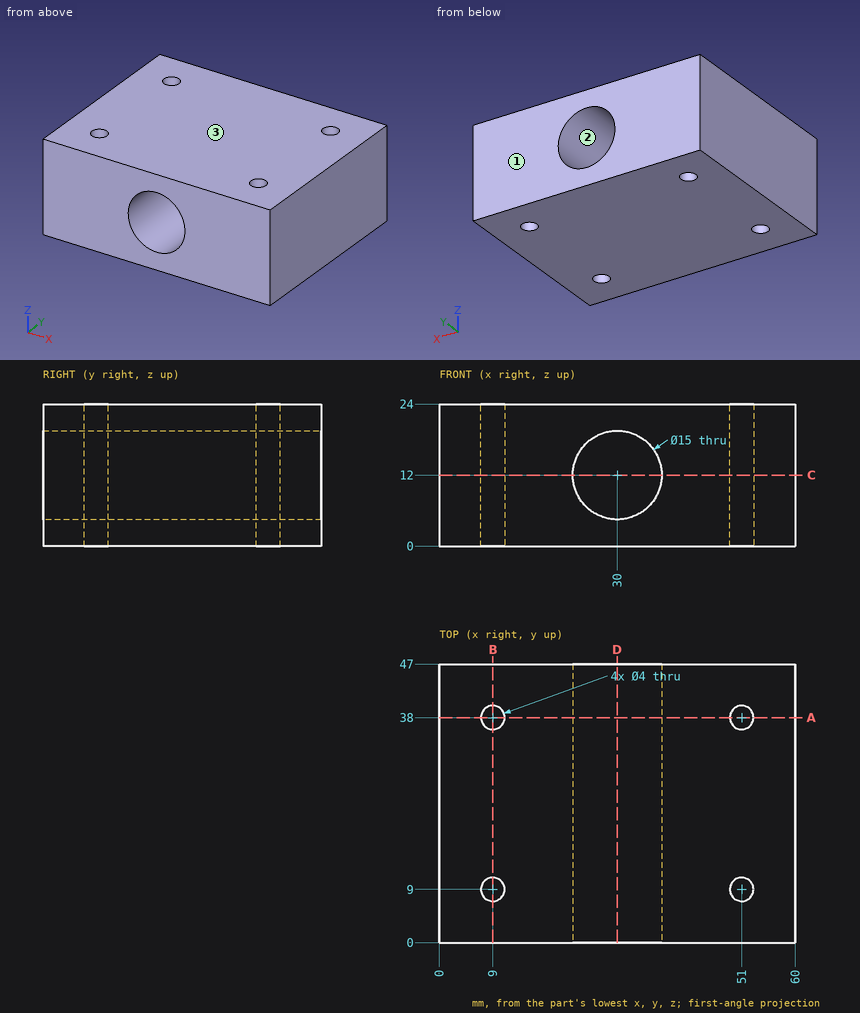
Input: dimensioned drawing with shaded views. Units: mm. Origin: part minimum x, y, z. Round coordinates to 2 decimals unless told otherwise and drop trailing zeros. Loops run counter-clockwise (first coordinate to the right, second up) from the corner with the lowest first, then second, coordinate; pieces in that order, holes last. Notation, with made-up numbers: M 66.25,88.5 L 115.25,88.5 A16 ccw 115.25,99.5 Z; hole C 9,8.5 d10. An arc over 180 degrees is marked long. One line per question, with ' | ' between items.
(1) Cut plane D-D on x = 30. Return the cut outline in (y, z), plus the area to 3 significant figures.
Check result:
outline: M 0,0 L 47,0 L 47,4.5 L 0,4.5 Z; M 0,19.5 L 47,19.5 L 47,24 L 0,24 Z | area: 423 mm2
(2) Cut plane C-C on z = 12. Return the cut outline in (x, y).
Check result:
outline: M 0,0 L 22.5,0 L 22.5,47 L 0,47 Z; M 37.5,0 L 60,0 L 60,47 L 37.5,47 Z; hole C 9,9 d4; hole C 9,38 d4; hole C 51,9 d4; hole C 51,38 d4
(3) Pull-direction query (Z, two-part tool) for the marked faces 1, 2 and 3; classes: +Z half, -Z half, draft (parallel to the pull), parting line (faces both ways), or undercut.
Check result:
face 1: draft | face 2: undercut | face 3: +Z half
(4) Contact query for a flat-ended pin moving along its axis: P1, Ø3.5, axis at x = 51, y = 9, coming from the -Z side. Output: stop coordinate, or through.
Check result:
P1: passes through
(5) Cut plane A-A on y = 38. Return the cut outline in (x, z).
Check result:
outline: M 0,0 L 7,0 L 7,24 L 0,24 Z; M 11,0 L 49,0 L 49,24 L 11,24 Z; M 53,0 L 60,0 L 60,24 L 53,24 Z; hole C 30,12 d15
(6) Cut plane B-B on x = 9. Return the cut outline in (y, z), plus the area to 3 significant figures.
Check result:
outline: M 0,0 L 7,0 L 7,24 L 0,24 Z; M 11,0 L 36,0 L 36,24 L 11,24 Z; M 40,0 L 47,0 L 47,24 L 40,24 Z | area: 936 mm2
(7) Material intervals for line 1 along Y through (x, z) = (9, 12.5); line 2 along Y through (x, z) = (49.5, 21.75); line 3 along Z through (x, y) = (24, 16), sorted ascending. Write a range as from..to.
Check result:
line 1: y = 0..7, 11..36, 40..47 | line 2: y = 0..7.68, 10.32..36.68, 39.32..47 | line 3: z = 0..7.5, 16.5..24
